The listing builds one solid part. Answer for the finished solid, in the listing's coordinates (mm). Face numbers are marked on the shaded views. A direction names the side the tool comes from. Coordinates: 2 decimals unless noted, no trailing zeros. Order: outer loops, then holes, each group sorted by start corner. A loop starts at its lowest first (then second) coordinate and runs counter-clockwise, first axis right, second up. Notation, with made-up numbers: (71.5, 58.25) -> (109.5, 58.25) arc R25 cw to (109.5, 87.25) -> close; hole circle Ø6 at (3, 42). An arc over 180 degrees is marked (long way). Answer in a Markdown table with one row per item. Add a question column.
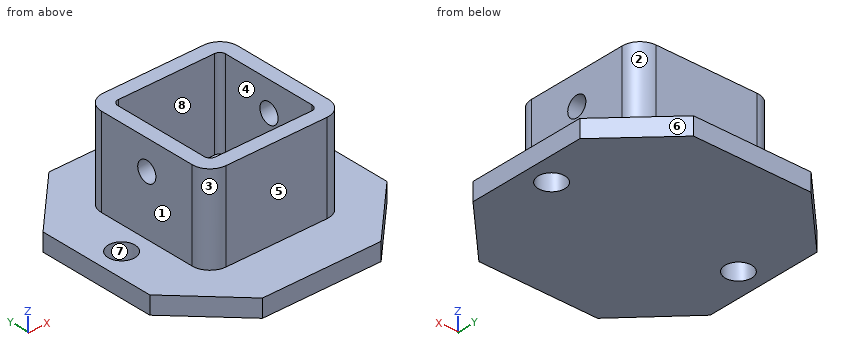
Autodesk Inventor part; units mm, degrees
ref_plane "YZ Plane" through (0, 0, 0) normal (1, 0, 0) x (0, 1, 0)
ref_plane "XZ Plane" through (0, 0, 0) normal (0, 1, 0) x (-1, 0, 0)
ref_plane "XY Plane" through (0, 0, 0) normal (0, 0, 1) x (1, 0, 0)
sketch "スケッチ1" plane through (0, 0, 0) normal (0, 0, 1) x (1, 0, 0)
  line L0 (-9.1, 9.1) -> (9.1, 9.1)
  line L1 (9.1, 9.1) -> (9.1, -9.1)
  line L2 (9.1, -9.1) -> (-9.1, -9.1)
  line L3 (-9.1, -9.1) -> (-9.1, 9.1)
  line L4 (-9.1, 9.1) -> (9.1, -9.1) construction
  line L5 (9.1, 9.1) -> (-9.1, -9.1) construction
  line L6 (-11.5, 11.5) -> (11.5, 11.5)
  line L7 (11.5, 11.5) -> (11.5, -11.5)
  line L8 (11.5, -11.5) -> (-11.5, -11.5)
  line L9 (-11.5, -11.5) -> (-11.5, 11.5)
  line L10 (-11.5, 11.5) -> (11.5, -11.5) construction
  line L11 (11.5, 11.5) -> (-11.5, -11.5) construction
  point P0 (0, 0)
  dimension "d0" = 18.2
  dimension "d1" = 18.2
  dimension "d2" = 23
  dimension "d3" = 23
extrude "押し出し1" add sketch "スケッチ1" along normal blind 15
sketch "スケッチ2" plane through (-11.5, -11.5, 0) normal (-1, 0, 0) x (0, 0, 1)
  circle A0 centre (10, 11.5) radius 1.7
  point P0 (0, 11.5)
  dimension "d6" = 3.4
extrude "押し出し2" cut sketch "スケッチ2" against normal blind 30
sketch "スケッチ3" plane through (0, 0, 0) normal (0, 0, -1) x (-1, 0, 0)
  line L0 (20, 20) -> (-20, 20)
  line L1 (-20, 20) -> (-20, -20)
  line L2 (-20, -20) -> (20, -20)
  line L3 (20, -20) -> (20, 20)
  line L4 (20, 20) -> (-20, -20) construction
  line L5 (-20, 20) -> (20, -20) construction
  point P0 (0, 0)
  dimension "d9" = 40
  dimension "d10" = 40
extrude "押し出し3" add sketch "スケッチ3" along normal blind 3
sketch "スケッチ4" plane through (0, 0, 0) normal (0, 0, 1) x (1, 0, 0)
  point P0 (0, 0)
sketch "スケッチ5" plane through (0, 0, 0) normal (0, 0, 1) x (1, 0, 0)
  circle A0 centre (-15.75, 0) radius 2.25
  circle A1 centre (15.75, 0) radius 2.25
  point P0 (0, 0)
  dimension "d13" = 4.5
  dimension "d14" = 4.5
extrude "押し出し4" cut sketch "スケッチ5" against normal blind 3
sketch "スケッチ6" plane through (0, 0, 0) normal (0, 0, 1) x (1, 0, 0)
  line L0 (-20, -20) -> (-20, 20)
  line L1 (-20, 20) -> (20, 20)
  line L2 (-20, 10) -> (-20, 20)
  line L3 (-20, 20) -> (-10, 20)
  line L4 (-10, 20) -> (-20, 10)
  line L5 (19.8208, 20) -> (9.8208, 20)
  line L6 (20, 20) -> (20, -20)
  line L7 (20, 20) -> (20, 10)
  line L8 (20, 10) -> (9.8208, 20)
  line L9 (-20, -20) -> (-20, -10)
  line L10 (-20, -20) -> (-10, -20)
  line L11 (20, -20) -> (-20, -20)
  line L12 (-10, -20) -> (-20, -10)
  line L13 (20, -20) -> (10, -20)
  line L14 (20, -20) -> (20, -10)
  line L15 (10, -20) -> (20, -10)
  point P0 (0, 0)
  dimension "d17" = 10
  dimension "d18" = 10
  dimension "d19" = 10
  dimension "d20" = 10
  dimension "d21" = 10
  dimension "d22" = 10
extrude "押し出し5" cut sketch "スケッチ6" against normal blind 3 contours L0 L12 L10 | L0 L1 L4 | L15 L6 L11 | L1 L6 L8
fillet "フィレット1" radius 3 4 edges at (-11.5, 11.5, 7.5) (11.5, 11.5, 7.5) (11.5, -11.5, 7.5) (-11.5, -11.5, 7.5)
fillet "フィレット2" radius 1 4 edges at (-9.1, 9.1, 7.5) (9.1, 9.1, 7.5) (-9.1, -9.1, 7.5) (9.1, -9.1, 7.5)
properties part number "rod_fixture_vp13"
Q1. Given pin 1 (9 mm diameter, centred on x = 0, y = -1, fed in from +Z); pin 2 (7.5 mm diameter, centred on x = -2, z = 8, fed in from -Y); pin 3 (1 mm diameter, centred on y = -3, z = 9, fed in from -X); pin 4 (3 mm diameter, centred on y = 0, z = 10, fed in from -X), each flat-ended and moving along its own axis, determine where each tip first touches the part or whether it passes through.
Q2. A cutting plane is placed at A-A (y = 0). Determine the outline of the cut face in (x, z).
Q3. A cutting plane is placed at C-C (z = 10). Determine the outline of the cut face in (x, y), then the cut area to 3 significant figures.
Q4. A cutting plane is placed at B-B (x = -15.75). Determine the outline of the cut face in (y, z).
Q5. For the marked faces 1, 2, 3 and 4, determine the directions among +Z, -Z, +X, -X, +Y, -Y from which every point of the face is accessible in a straight line to the end or side of a thin tool.
Q6. Straight lines are drawn through the part: line 1 (X direction, y = 3, z = 4.25); line 2 (Z direction, x = -2, y = 15.5). For each, find the intervals that lie inside material, in ascending order.
Q7. A cutting plane is placed at D-D (z = 14.25). Determine the outline of the cut face in (x, y), then the cut area to 3 significant figures.
Q8. Determine the mould class of the marked faces 5, 6, 7 and 8 for opening direction Y: +Y half, -Y half, draft (parallel to the pull), parting line (faces both ways), or undercut.
Returned:
| question | item | result |
|---|---|---|
| 1 | pin 1 | stops at z = 0 |
| 1 | pin 2 | stops at y = -11.5 |
| 1 | pin 3 | stops at x = -11.5 |
| 1 | pin 4 | passes through |
| 2 | outline | (-20, -3) -> (-18, -3) -> (-18, 0) -> (-20, 0) -> close; (-13.5, -3) -> (13.5, -3) -> (13.5, 0) -> (11.5, 0) -> (11.5, 8.3) -> (9.1, 8.3) -> (9.1, 0) -> (-9.1, 0) -> (-9.1, 8.3) -> (-11.5, 8.3) -> (-11.5, 0) -> (-13.5, 0) -> close; (-11.5, 11.7) -> (-9.1, 11.7) -> (-9.1, 15) -> (-11.5, 15) -> close; (9.1, 11.7) -> (11.5, 11.7) -> (11.5, 15) -> (9.1, 15) -> close; (18, -3) -> (20, -3) -> (20, 0) -> (18, 0) -> close |
| 3 | outline | (-11.5, -8.5) arc R3 ccw to (-8.5, -11.5) -> (8.5, -11.5) arc R3 ccw to (11.5, -8.5) -> (11.5, -1.7) -> (9.1, -1.7) -> (9.1, -8.1) arc R1 cw to (8.1, -9.1) -> (-8.1, -9.1) arc R1 cw to (-9.1, -8.1) -> (-9.1, -1.7) -> (-11.5, -1.7) -> close; (-11.5, 1.7) -> (-9.1, 1.7) -> (-9.1, 8.1) arc R1 cw to (-8.1, 9.1) -> (8.1, 9.1) arc R1 cw to (9.1, 8.1) -> (9.1, 1.7) -> (11.5, 1.7) -> (11.5, 8.5) arc R3 ccw to (8.5, 11.5) -> (-8.5, 11.5) arc R3 ccw to (-11.5, 8.5) -> close |
| 3 | area | 175 mm² |
| 4 | outline | (-14.25, -3) -> (-2.25, -3) -> (-2.25, 0) -> (-14.25, 0) -> close; (2.25, -3) -> (14.25, -3) -> (14.25, 0) -> (2.25, 0) -> close |
| 5 | face 1 | +Z, -X, +Y, -Y |
| 5 | face 2 | +Z, +X, +Y |
| 5 | face 3 | +Z, -X, -Y |
| 5 | face 4 | +Z |
| 6 | line 1 | x = -11.5 to -9.1, 9.1 to 11.5 |
| 6 | line 2 | z = -3 to 0 |
| 7 | outline | (-11.5, -8.5) arc R3 ccw to (-8.5, -11.5) -> (8.5, -11.5) arc R3 ccw to (11.5, -8.5) -> (11.5, 8.5) arc R3 ccw to (8.5, 11.5) -> (-8.5, 11.5) arc R3 ccw to (-11.5, 8.5) -> close; hole (-9.1, -8.1) arc R1 ccw to (-8.1, -9.1) -> (8.1, -9.1) arc R1 ccw to (9.1, -8.1) -> (9.1, 8.1) arc R1 ccw to (8.1, 9.1) -> (-8.1, 9.1) arc R1 ccw to (-9.1, 8.1) -> close |
| 7 | area | 191 mm² |
| 8 | face 5 | -Y half |
| 8 | face 6 | +Y half |
| 8 | face 7 | undercut |
| 8 | face 8 | undercut |
